The model under review builds one solid part; all positions refer to its coordinate system, in mm. Give positions to 0.01 mm unless a question says otherwise; leave off trailing zeros. Put each result on its own line as item: value.
```python
from build123d import *

# Parameters (mm, degrees)
F0_R     = 2.1
F1_DEPTH = 505


with BuildPart() as f1:
    # F0 (on Top) → F1 (new body)
    with BuildSketch(Plane.XY):
        with BuildLine():
            Line((4.64, -10), (8.5, -10))
            Line((8.5, -10), (11.5, -10))
            Line((11.5, -10), (15.36, -10))
            Line((15.36, -10), (17.16, -8.2))
            Line((17.16, -8.2), (14.50066, -8.2))
            Line((14.50066, -8.2), (14.50066, -6.56))
            Line((14.50066, -6.56), (17.16, -3.90066))
            Line((17.16, -3.90066), (19.75, -3.90066))
            Line((19.75, -3.90066), (20, -3.65066))
            Line((20, -3.65066), (20.25, -3.90066))
            Line((20.25, -3.90066), (22.84, -3.90066))
            Line((22.84, -3.90066), (25.49934, -6.56))
            Line((25.49934, -6.56), (25.49934, -8.2))
            Line((25.49934, -8.2), (22.84, -8.2))
            Line((22.84, -8.2), (24.64, -10))
            Line((24.64, -10), (28.5, -10))
            ThreePointArc((28.5, -10), (29.56066, -9.56066), (30, -8.5))
            Line((30, -8.5), (30, -4.64))
            Line((30, -4.64), (28.2, -2.84))
            Line((28.2, -2.84), (28.2, -5.49934))
            Line((28.2, -5.49934), (26.56, -5.49934))
            Line((26.56, -5.49934), (23.90066, -2.84))
            Line((23.90066, -2.84), (23.90066, -0.25))
            Line((23.90066, -0.25), (23.65066, 0))
            Line((23.65066, 0), (23.90066, 0.25))
            Line((23.90066, 0.25), (23.90066, 2.84))
            Line((23.90066, 2.84), (26.56, 5.49934))
            Line((26.56, 5.49934), (28.2, 5.49934))
            Line((28.2, 5.49934), (28.2, 2.84))
            Line((28.2, 2.84), (30, 4.64))
            Line((30, 4.64), (30, 8.5))
            ThreePointArc((30, 8.5), (29.56066, 9.56066), (28.5, 10))
            Line((28.5, 10), (24.64, 10))
            Line((24.64, 10), (22.84, 8.2))
            Line((22.84, 8.2), (25.49934, 8.2))
            Line((25.49934, 8.2), (25.49934, 6.56))
            Line((25.49934, 6.56), (22.84, 3.90066))
            Line((22.84, 3.90066), (20.25, 3.90066))
            Line((20.25, 3.90066), (20, 3.65066))
            Line((20, 3.65066), (19.75, 3.90066))
            Line((19.75, 3.90066), (17.16, 3.90066))
            Line((17.16, 3.90066), (14.50066, 6.56))
            Line((14.50066, 6.56), (14.50066, 8.2))
            Line((14.50066, 8.2), (17.16, 8.2))
            Line((17.16, 8.2), (15.36, 10))
            Line((15.36, 10), (11.5, 10))
            Line((11.5, 10), (8.5, 10))
            Line((8.5, 10), (4.64, 10))
            Line((4.64, 10), (2.84, 8.2))
            Line((2.84, 8.2), (5.49934, 8.2))
            Line((5.49934, 8.2), (5.49934, 6.56))
            Line((5.49934, 6.56), (2.84, 3.90066))
            Line((2.84, 3.90066), (0.25, 3.90066))
            Line((0.25, 3.90066), (0, 3.65066))
            Line((0, 3.65066), (-0.25, 3.90066))
            Line((-0.25, 3.90066), (-2.84, 3.90066))
            Line((-2.84, 3.90066), (-5.49934, 6.56))
            Line((-5.49934, 6.56), (-5.49934, 8.2))
            Line((-5.49934, 8.2), (-2.84, 8.2))
            Line((-2.84, 8.2), (-4.64, 10))
            Line((-4.64, 10), (-8.5, 10))
            ThreePointArc((-8.5, 10), (-9.56066, 9.56066), (-10, 8.5))
            Line((-10, 8.5), (-10, 4.64))
            Line((-10, 4.64), (-8.2, 2.84))
            Line((-8.2, 2.84), (-8.2, 5.49934))
            Line((-8.2, 5.49934), (-6.56, 5.49934))
            Line((-6.56, 5.49934), (-3.90066, 2.84))
            Line((-3.90066, 2.84), (-3.90066, 0.25))
            Line((-3.90066, 0.25), (-3.65066, 0))
            Line((-3.65066, 0), (-3.90066, -0.25))
            Line((-3.90066, -0.25), (-3.90066, -2.84))
            Line((-3.90066, -2.84), (-6.56, -5.49934))
            Line((-6.56, -5.49934), (-8.2, -5.49934))
            Line((-8.2, -5.49934), (-8.2, -2.84))
            Line((-8.2, -2.84), (-10, -4.64))
            Line((-10, -4.64), (-10, -8.5))
            ThreePointArc((-10, -8.5), (-9.56066, -9.56066), (-8.5, -10))
            Line((-8.5, -10), (-4.64, -10))
            Line((-4.64, -10), (-2.84, -8.2))
            Line((-2.84, -8.2), (-5.49934, -8.2))
            Line((-5.49934, -8.2), (-5.49934, -6.56))
            Line((-5.49934, -6.56), (-2.84, -3.90066))
            Line((-2.84, -3.90066), (-0.25, -3.90066))
            Line((-0.25, -3.90066), (0, -3.65066))
            Line((0, -3.65066), (0.25, -3.90066))
            Line((0.25, -3.90066), (2.84, -3.90066))
            Line((2.84, -3.90066), (5.49934, -6.56))
            Line((5.49934, -6.56), (5.49934, -8.2))
            Line((5.49934, -8.2), (2.84, -8.2))
            Line((2.84, -8.2), (4.64, -10))
        make_face()
        Polygon((-6.56934, -7.63), (-6.56934, -8.2), (-8.2, -8.2), (-8.2, -6.56934), (-7.63, -6.56934), align=None, mode=Mode.SUBTRACT)
        Polygon((27.63, -6.56934), (28.2, -6.56934), (28.2, -8.2), (26.56934, -8.2), (26.56934, -7.63), align=None, mode=Mode.SUBTRACT)
        Circle(F0_R, mode=Mode.SUBTRACT)
        Polygon((-7.63, 6.56934), (-8.2, 6.56934), (-8.2, 8.2), (-6.56934, 8.2), (-6.56934, 7.63), align=None, mode=Mode.SUBTRACT)
        Polygon((3.90066, 2.84), (6.56, 5.49934), (6.99934, 5.93868), (6.99934, 8.2), (13.00066, 8.2), (13.00066, 5.93868), (13.44, 5.49934), (16.09934, 2.84), (16.09934, 0.25), (16.34934, 0), (16.09934, -0.25), (16.09934, -2.84), (13.44, -5.49934), (13.00066, -5.93868), (13.00066, -8.2), (6.99934, -8.2), (6.99934, -5.93868), (6.56, -5.49934), (3.90066, -2.84), (3.90066, -0.25), (3.65066, 0), (3.90066, 0.25), align=None, mode=Mode.SUBTRACT)
        with Locations((20, 0)):
            Circle(F0_R, mode=Mode.SUBTRACT)
        Polygon((28.2, 8.2), (28.2, 6.56934), (27.63, 6.56934), (26.56934, 7.63), (26.56934, 8.2), align=None, mode=Mode.SUBTRACT)
    extrude(amount=F1_DEPTH)


solid = f1.part
```
(1) Take a section at A-A, the plane z = 223.5. Count the separate pieces of the cut face and the enclosed holes in it, then the cut area to 3 significant figures.
The answers:
separate pieces: 1
enclosed holes: 7
area: 287 mm^2
(2) Wall thickness on L1, parallel to Y at x = 28, z = 150.5; L2, parallel to X at y = 4.75, z = 447; L3, parallel to Y at x = 20, z = 200: over which ranges is each line inside the solid? List them lowest first.
The answers:
L1: -10 to -8.2, -6.57 to -5.5, 5.5 to 6.57, 8.2 to 10
L2: -10 to -8.2, -5.81 to -3.69, 3.69 to 5.81, 14.19 to 16.31, 23.69 to 25.81, 28.2 to 30
L3: -3.65 to -2.1, 2.1 to 3.65
(3) Clearance check with flat-ended pins moving along their axes: pin 1 Ø3 at (x, z) = (21.5, 300.5) entering from +Y; pin 2 Ø3 at (x, z) = (18.5, 378) entering from -Y; pin 3 Ø0.8 at (x, z) = (24, 367) entering from +Y; pin 4 Ø3.5 at (x, y) = (0, 0) entering from +Z. State where each tip first meets the part, or that it passes through.
The answers:
pin 1: y = 8.36
pin 2: y = -8.36
pin 3: y = 9.76
pin 4: through
